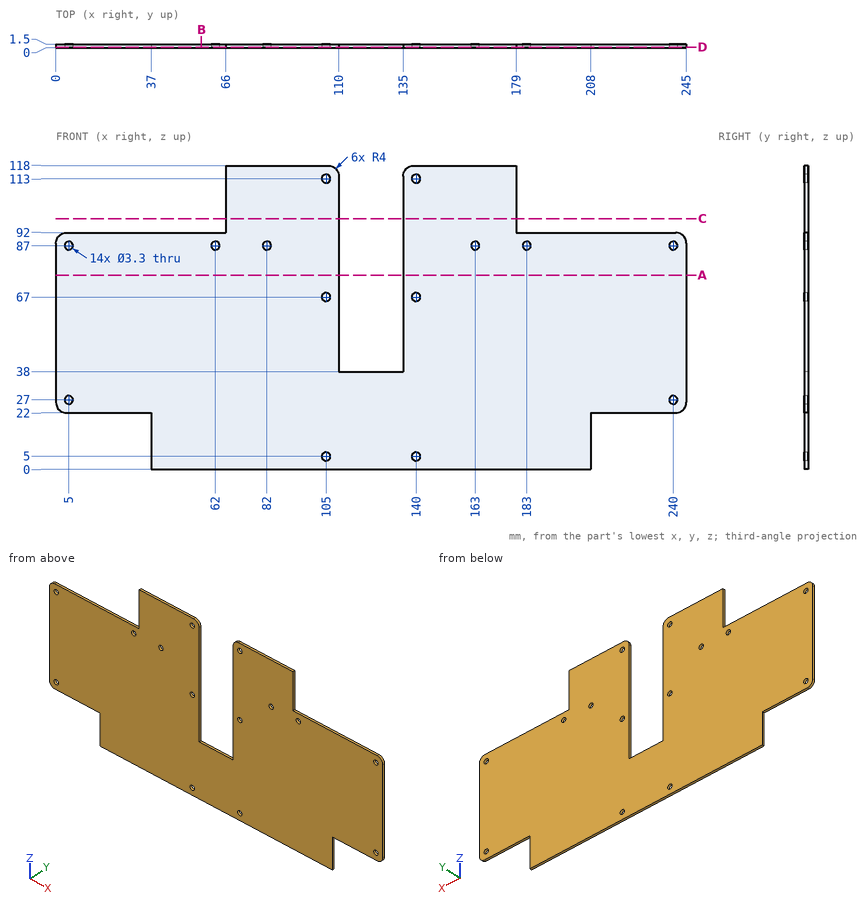
Check sheet for the drawn part. Datum: minimum x, y, z corner. Units: mm. Coordinates: 2 decimals unless noted, no trailing zeros. Loops run counter-clockwise (first coordinate to the right, second up) from the corner with the lowest first, then second, coordinate; pieces in that order, holes last. Notation, with made-up numbers: M -28.75,89 L 30.25,89 A7 cw 30.25,96 Z; hole C 6.5,19 d5. An arc over 180 degrees is marked long. Answer as a JSON object with one key per item and string values.
1. Sectioned sample at B-B on x = 56.5. Record the cut outline in (y, z).
Outcome:
{"outline": "M 0,0 L 1.5,0 L 1.5,92 L 0,92 Z"}
2. Scan lines: L1, parallel to Z at x = 5, y = 1.1; L2, parallel to X at y = 0.9, z = 67; L3, parallel to X at y = 0.8, z = 81. Record each from-to range of solid material in increasing order. Write a range as from..to.
Outcome:
{"L1": "22..25.35, 28.65..85.35, 88.65..92", "L2": "0..103.35, 106.65..110, 135..138.35, 141.65..245", "L3": "0..110, 135..245"}
3. Sectioned sample at D-D on y = 0.25. Count the separate pieces of the cut face and the enclosed holes in it, and give its area (3 significant figures).
Outcome:
{"separate pieces": "1", "enclosed holes": "14", "area": "21,700 mm²"}
4. Depth check by flat-ended pin: P1, Ø2.5, axis at x = 140, z = 5, coming from the -Y side; P2, Ø0.8, axis at y = 0.5, z = 6, coming from the +X side; P3, Ø0.8, axis at x = 214.5, y = 1, coming from the +Z side. Enter the tip coordinate at first touch or a pass-through.
Outcome:
{"P1": "through", "P2": "x = 208", "P3": "z = 92"}
5. Sectioned sample at A-A on z = 75.5. Record the cut outline in (x, y), and give its area (3 significant figures).
Outcome:
{"outline": "M 0,0 L 110,0 L 110,1.5 L 0,1.5 Z; M 135,0 L 245,0 L 245,1.5 L 135,1.5 Z", "area": "330 mm²"}
6. Sectioned sample at C-C on z = 97.5. Record the cut outline in (x, y), and give its area (3 significant figures).
Outcome:
{"outline": "M 66,0 L 110,0 L 110,1.5 L 66,1.5 Z; M 135,0 L 179,0 L 179,1.5 L 135,1.5 Z", "area": "132 mm²"}
